Work out the finished part from the listing and answer in its coordinate system (mm). Face numbers are marked on the shaded views. A direction names the side the tool comes from. Round coordinates to 2 decimals unless told otherwise and drop trailing zeros. Write each loop counter-clockwise with the first axis right and the second up, starting at its lowest first coordinate (ties: lowest second). Pieces come first, ordered by that corner, then holes.
1. Find section B-B (x = -13). Write down the section's boundary in (y, z).
2. Determine the mould class of the marked faces 1, 2 and 3 for opening direction Y: pulls with the +Y half, pulls with the -Y half, needs draft (parallel to the pull), parting line crosses it, or undercut.
3. Find section A-A (y = 74.5). Write down the section's boundary in (x, z).
4. Find section C-C (z = 39.5). Write down the section's boundary in (x, y), and give its area (3 significant figures).
5. Find section D-D (x = -6). Write down the section's boundary in (y, z), and give its area (3 significant figures).
6. Flat-ended cylindrical pins translate along their axes: pin 1 Ø8 at (x, z) = (-12, 35.5) entering from -Y; pin 2 Ø3.5 at (y, z) = (49, 31.5) entering from -X; pin 3 Ø9 at (x, y) = (-8.5, 77.5) entering from +Z; pin 4 Ø3 at (x, z) = (-6, 29.49) entering from -Y. Find the tip coordinate at first contact, or state that the pin passes through.
7. A tool of negligible diameter and unlimited length cuts with its end or side. For the marked faces 4, 5, 6 and 7, from which of +Z, -Z, +X, -X, +Y, -Y can it reach the whole face along a straight path? Write none if from no direction.
8. Straight lines are drawn through the part: probe 1 along X at (y, z) = (54, 35); probe 2 along Z at (x, y) = (-7.5, 89); probe 3 along Y at (x, z) = (-2.75, 32.25). For each, find the intervals that lie inside material, in ascending order.
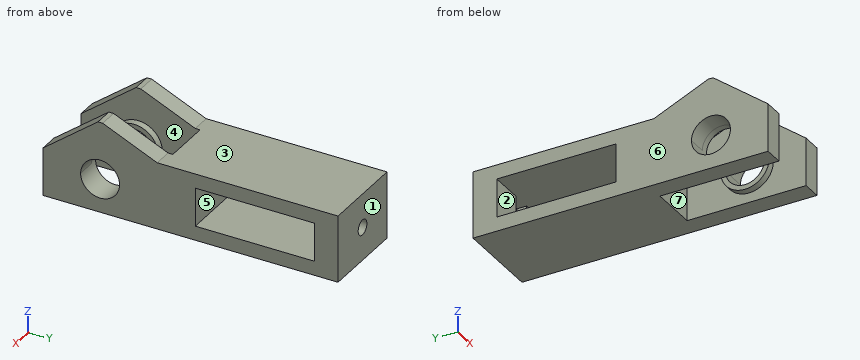
```python
from build123d import *

# Parameters (mm, degrees)
SKETCH_R        = 4.1
SKETCH_W        = 25
SKETCH_H        = 8.1
PAD_DEPTH       = 18
SKETCH001_W     = 25
SKETCH001_H     = 10
POCKET_DEPTH    = 25
SKETCH002_R     = 5.1
SKETCH002_R_2   = 4.1
PAD001_DEPTH    = 18
SKETCH003_W     = 24
SKETCH003_H     = 7
POCKET001_DEPTH = 25
SKETCH004_R     = 1.6
POCKET002_DEPTH = 5
SKETCH005_W     = 8.1
SKETCH005_H     = 4
POCKET003_DEPTH = 2
POCKET004_DEPTH = 25


with BuildPart() as part:
    # Sketch → Pad (new body)
    with BuildSketch(Plane(origin=(-15, 105, 17), x_dir=(0, 1, 0), z_dir=(1, 0, 0))):
        Polygon((-68.082832, 24.585315), (-44.082832, 24.585315), (-44.082832, 19.585315), (-6.082832, 19.585315), (-6.082832, 5.485315), (-68.082832, 5.485315), align=None)
        with Locations((-56.082832, 12.485315)):
            Circle(SKETCH_R, mode=Mode.SUBTRACT)
        with Locations((-23.582832, 12.535315)):
            Rectangle(SKETCH_W, SKETCH_H, mode=Mode.SUBTRACT)
    extrude(amount=PAD_DEPTH)

    # Sketch001 → Pocket (cut)
    with BuildSketch(Plane(origin=(-15, 105, 41.585315), x_dir=(0, -1, 0), z_dir=(0, 0, 1))):
        with Locations((55.582832, 9)):
            Rectangle(SKETCH001_W, SKETCH001_H)
    extrude(amount=-POCKET_DEPTH, mode=Mode.SUBTRACT)

    # Sketch002 → Pad001 (new body)
    with BuildSketch(Plane(origin=(3, 105, 17), x_dir=(0, 1, 0), z_dir=(1, 0, 0))):
        with Locations((-56.082832, 12.585315)):
            Circle(SKETCH002_R)
        with Locations((-56.082832, 12.585315)):
            Circle(SKETCH002_R_2, mode=Mode.SUBTRACT)
    extrude(amount=-PAD001_DEPTH)

    # Sketch003 → Pocket001 (cut)
    with BuildSketch(Plane(origin=(-15, 105, 36.585315), x_dir=(0, -1, 0), z_dir=(0, 0, 1))):
        with Locations((55.082832, 9)):
            Rectangle(SKETCH003_W, SKETCH003_H)
    extrude(amount=-POCKET001_DEPTH, mode=Mode.SUBTRACT)

    # Sketch004 → Pocket002 (cut)
    with BuildSketch(Plane(origin=(-15, 98.917168, 17), x_dir=(0, 0, 1), z_dir=(0, 1, 0))):
        with Locations((12.485315, 9)):
            Circle(SKETCH004_R)
    extrude(amount=-POCKET002_DEPTH, mode=Mode.SUBTRACT)

    # Sketch005 → Pocket003 (cut)
    with BuildSketch(Plane(origin=(-15, 93.917168, 17), x_dir=(0, 0, -1), z_dir=(0, -1, 0))):
        with Locations((-12.535315, 9)):
            Rectangle(SKETCH005_W, SKETCH005_H)
    extrude(amount=-POCKET003_DEPTH, mode=Mode.SUBTRACT)

    # Sketch006 → Pocket004 (cut)
    with BuildSketch(Plane(origin=(3, 105, 17), x_dir=(0, 1, 0), z_dir=(1, 0, 0))):
        Polygon((-55.529856, 24.585315), (-44.082832, 19.585315), (-44.082832, 24.585315), align=None)
        Polygon((-56.529856, 24.585315), (-68.082832, 15.585315), (-68.082832, 24.585315), align=None)
    extrude(amount=-POCKET004_DEPTH, mode=Mode.SUBTRACT)


solid = part.part
```
Worked answers:
1. outline: (36.92, 22.49) - (98.92, 22.49) - (98.92, 36.59) - (60.92, 36.59) - (49.47, 41.59) - (48.47, 41.59) - (36.92, 32.59) - close; hole (44.82, 29.54) arc R4.1 ccw to (53.02, 29.54) arc R4.1 ccw to start; hole (68.92, 25.49) - (93.92, 25.49) - (93.92, 33.59) - (68.92, 33.59) - close
2. face 1: pulls with the +Y half
2. face 2: undercut
2. face 3: needs draft
3. outline: (-15, 22.49) - (3, 22.49) - (3, 25.49) - (-15, 25.49) - close; (-15, 33.59) - (3, 33.59) - (3, 36.59) - (-15, 36.59) - close
4. outline: (-15, 45.79) - (-11, 45.79) - (-11, 54.24) - (-15, 54.24) - close; (-1, 45.79) - (3, 45.79) - (3, 54.24) - (-1, 54.24) - close
4. area: 67.6 mm2
5. outline: (61.92, 22.49) - (98.92, 22.49) - (98.92, 27.89) - (95.92, 27.89) - (95.92, 25.49) - (68.92, 25.49) - (68.92, 33.59) - (95.92, 33.59) - (95.92, 31.09) - (98.92, 31.09) - (98.92, 36.59) - (61.92, 36.59) - close
5. area: 293 mm2
6. pin 1: stops at y = 36.92
6. pin 2: passes through
6. pin 3: stops at z = 36.59
6. pin 4: stops at y = 61.92
7. face 4: none
7. face 5: +X, -X
7. face 6: +Z, -Z, -X, +Y, -Y
7. face 7: +Z, -Z
8. probe 1: x = -15 to -11, -1 to 3
8. probe 2: z = 22.49 to 25.49, 33.59 to 36.59
8. probe 3: y = 61.92 to 68.92, 93.92 to 98.92
